from build123d import *

# Parameters (mm, degrees)
F0_R      = 2.413
F1_DEPTH  = 8
F2_W      = 69.36
F2_H      = 50.39
F3_DEPTH  = 25.4
F4_W      = 69.36
F4_H      = 50.39
F5_DEPTH  = 2.35
F6_DEPTH  = 2
F7_R      = 5
F8_DEPTH  = 6
F9_R      = 3.625
F10_DEPTH = 25.4
F11_R     = 3.625
F12_DEPTH = 25.4
F13_R     = 3.625
F14_DEPTH = 25.4
F15_R     = 2.413
F15_R_2   = 5
F15_W     = 71.86
F15_H     = 55.89
F16_DEPTH = 2
F17_W     = 36.8478260934
F17_H     = 40.4230296794
F18_DEPTH = 6


with BuildPart() as f1:
    # F0 (on Top) → F1 (new body)
    with BuildSketch(Plane.XY):
        with BuildLine():
            ThreePointArc((-69.85, 36.195), (-75.2381536726, 33.9631536726), (-77.47, 28.575))
            Line((-77.47, 28.575), (-77.47, 0))
            Line((-77.47, 0), (-77.47, -28.575))
            ThreePointArc((-77.47, -28.575), (-75.2381536726, -33.9631536726), (-69.85, -36.195))
            Line((-69.85, -36.195), (0, -36.195))
            Line((0, -36.195), (69.85, -36.195))
            ThreePointArc((69.85, -36.195), (75.2381536726, -33.9631536726), (77.47, -28.575))
            Line((77.47, -28.575), (77.47, 0))
            Line((77.47, 0), (77.47, 28.575))
            ThreePointArc((77.47, 28.575), (75.2381536726, 33.9631536726), (69.85, 36.195))
            Line((69.85, 36.195), (0, 36.195))
            Line((0, 36.195), (-69.85, 36.195))
        make_face()
        with Locations((-69.85, -28.575)):
            Circle(F0_R, mode=Mode.SUBTRACT)
        with Locations((69.85, -28.575)):
            Circle(F0_R, mode=Mode.SUBTRACT)
        with Locations((-69.85, 28.575)):
            Circle(F0_R, mode=Mode.SUBTRACT)
        with Locations((69.85, 28.575)):
            Circle(F0_R, mode=Mode.SUBTRACT)
    extrude(amount=F1_DEPTH)

    # F2 (on face) → F3 (cut)
    with BuildSketch(Plane(origin=(0, 0, 0), x_dir=(1, 0, 0), z_dir=(0, 0, -1))):
        with Locations((-23.74, 0.000232)):
            Rectangle(F2_W, F2_H)
    extrude(amount=-F3_DEPTH, mode=Mode.SUBTRACT)

    # F4 (on face) → F5 (cut)
    with BuildSketch(Plane.XY.offset(8)):
        with Locations((-23.74, -0.000232)):
            Rectangle(F4_W, F4_H)
        Polygon((-58.42, -25.195232), (-58.42, -27.695232), (13.44, -27.695232), (13.44, 28.194768), (-58.42, 28.194768), (-58.42, 25.194768), (10.94, 25.194768), (10.94, -25.195232), align=None)
    extrude(amount=-F5_DEPTH, mode=Mode.SUBTRACT)

    # F6 (add): a face of the model
    f6_faces = [f1.faces().sort_by_distance(p)[0] for p in [
        (-74.0288829068, 32.7538829068, 8),
    ]]
    extrude(f6_faces, amount=F6_DEPTH)

    # F7 (on face) → F8 (cut)
    with BuildSketch(Plane.XY.offset(10)):
        with Locations((62.47, -20)):
            Circle(F7_R)
        with Locations((42.47, -20)):
            Circle(F7_R)
        with Locations((62.47, 0)):
            Circle(F7_R)
    extrude(amount=-F8_DEPTH, mode=Mode.SUBTRACT)

    # F9 (on face) → F10 (cut)
    with BuildSketch(Plane.XY.offset(4)):
        with Locations((62.47, 0)):
            Circle(F9_R)
    extrude(amount=-F10_DEPTH, mode=Mode.SUBTRACT)

    # F11 (on face) → F12 (cut)
    with BuildSketch(Plane.XY.offset(4)):
        with Locations((62.47, -20)):
            Circle(F11_R)
    extrude(amount=-F12_DEPTH, mode=Mode.SUBTRACT)

    # F13 (on face) → F14 (cut)
    with BuildSketch(Plane.XY.offset(4)):
        with Locations((42.47, -20)):
            Circle(F13_R)
    extrude(amount=-F14_DEPTH, mode=Mode.SUBTRACT)

    # F15 (on face) → F16 (cut)
    with BuildSketch(Plane.XY.offset(10)):
        with BuildLine():
            Line((69.85, 36.195), (-69.85, 36.195))
            ThreePointArc((-69.85, 36.195), (-75.2381536726, 33.9631536726), (-77.47, 28.575))
            Line((-77.47, 28.575), (-77.47, -28.575))
            ThreePointArc((-77.47, -28.575), (-75.2381536726, -33.9631536726), (-69.85, -36.195))
            Line((-69.85, -36.195), (69.85, -36.195))
            ThreePointArc((69.85, -36.195), (75.2381536726, -33.9631536726), (77.47, -28.575))
            Line((77.47, -28.575), (77.47, 28.575))
            ThreePointArc((77.47, 28.575), (75.2381536726, 33.9631536726), (69.85, 36.195))
        make_face()
        with Locations((-69.85, -28.575)):
            Circle(F15_R, mode=Mode.SUBTRACT)
        with Locations((69.85, -28.575)):
            Circle(F15_R, mode=Mode.SUBTRACT)
        with Locations((42.47, -20)):
            Circle(F15_R_2, mode=Mode.SUBTRACT)
        with Locations((62.47, -20)):
            Circle(F15_R_2, mode=Mode.SUBTRACT)
        with Locations((-22.49, 0.249768)):
            Rectangle(F15_W, F15_H, mode=Mode.SUBTRACT)
        with Locations((-69.85, 28.575)):
            Circle(F15_R, mode=Mode.SUBTRACT)
        with Locations((62.47, 0)):
            Circle(F15_R_2, mode=Mode.SUBTRACT)
        with Locations((69.85, 28.575)):
            Circle(F15_R, mode=Mode.SUBTRACT)
    extrude(amount=-F16_DEPTH, mode=Mode.SUBTRACT)

    # F17 (on face) → F18 (cut)
    with BuildSketch(Plane.XY.offset(8)):
        with Locations((36.5217383951, 7.9832531603)):
            Rectangle(F17_W, F17_H)
    extrude(amount=-F18_DEPTH, mode=Mode.SUBTRACT)


solid = f1.part
The listing builds one solid part. Answer for the finished solid, in the listing's coordinates (mm). A direction names the side the tool comes from. Give positions to 0.01 mm unless a question says otherwise; leave off trailing zeros. Loops run counter-clockwise (first coordinate to the right, second up) from the corner with the lowest first, then second, coordinate; pieces in that order, holes last.
Item 1: A tool of negligible diameter and unlimited length cuts with its end or side. For faces 4 (the flat face through (46, -18, 4)), 5 (the flat face through (10.94, 0, 3)), 6 (the flat face through (16, 1, 0)), from which of +Z, -Z, +X, -X, +Y, -Y can it reach the whole face along a straight path? Write none if from no direction.
Derived:
face 4: +Z
face 5: +Z, -Z
face 6: -Z, +X, -X, +Y, -Y
Item 2: A cutting plane is placed at A-A (y = 8.5). Give the vertices of the cut face in (x, z).
Derived:
outline: (-77.47, 0) - (-58.42, 0) - (-58.42, 8) - (-77.47, 8) - close; (10.94, 0) - (77.47, 0) - (77.47, 8) - (54.95, 8) - (54.95, 2) - (18.1, 2) - (18.1, 8) - (13.44, 8) - (13.44, 5.65) - (10.94, 5.65) - close
Item 3: A cutting plane is placed at D-D (x = 62.47). Give the vertices of the cut face in (y, z) (3 decimals).
Derived:
outline: (-36.195, 0) - (-23.625, 0) - (-23.625, 4) - (-25, 4) - (-25, 8) - (-36.195, 8) - close; (-16.375, 0) - (-3.625, 0) - (-3.625, 4) - (-5, 4) - (-5, 8) - (-15, 8) - (-15, 4) - (-16.375, 4) - close; (3.625, 0) - (36.195, 0) - (36.195, 8) - (5, 8) - (5, 4) - (3.625, 4) - close
Item 4: Find the intervals of material crossed by line 1 along Y through (x, z) = (69.85, 6.25) (3 decimals); line 2 along X through (y, z) = (-10, 3.25); line 3 along X through (y, z) = (-1, 1.5), in increasing order.
Derived:
line 1: y = -36.195 to -30.988, -26.162 to 26.162, 30.988 to 36.195
line 2: x = -77.47 to -58.42, 10.94 to 18.1, 54.95 to 77.47
line 3: x = -77.47 to -58.42, 10.94 to 58.99, 65.95 to 77.47
Item 5: A cutting plane is placed at B-B (y = 0). Give the vertices of the cut face in (x, z) (3 decimals).
Derived:
outline: (-77.47, 0) - (-58.42, 0) - (-58.42, 8) - (-77.47, 8) - close; (10.94, 0) - (58.845, 0) - (58.845, 4) - (57.47, 4) - (57.47, 8) - (54.946, 8) - (54.946, 2) - (18.098, 2) - (18.098, 8) - (13.44, 8) - (13.44, 5.65) - (10.94, 5.65) - close; (66.095, 0) - (77.47, 0) - (77.47, 8) - (67.47, 8) - (67.47, 4) - (66.095, 4) - close
Item 6: Determine the mould class of faces 1 (the flat face through (-1, -36.195, 4)), 2 (the flat face through (-77.47, 0, 4)), 3 (the flat face through (36, -12.228, 5)) for opening direction Y: +Y half, -Y half, draft (parallel to the pull), parting line (faces both ways), or undercut.
Derived:
face 1: -Y half
face 2: draft
face 3: undercut
Item 7: Each of these flat-tipped pins is pushed along its axis until it touches: pin 1 Ø6 at (x, y) = (62.47, 0) entering from -Z; pin 2 Ø18.5 at (x, y) = (30, 1) entering from +Z. Where does it stop, or does it pass through?
Derived:
pin 1: passes through
pin 2: stops at z = 2
Item 8: A cutting plane is placed at C-C (x = 42.47). Give the vertices of the cut face in (y, z) (3 decimals), then the cut area to 3 significant figures.
Derived:
outline: (-36.195, 0) - (-23.625, 0) - (-23.625, 4) - (-25, 4) - (-25, 8) - (-36.195, 8) - close; (-16.375, 0) - (36.195, 0) - (36.195, 8) - (28.195, 8) - (28.195, 2) - (-12.228, 2) - (-12.228, 8) - (-15, 8) - (-15, 4) - (-16.375, 4) - close
area: 268 mm2
